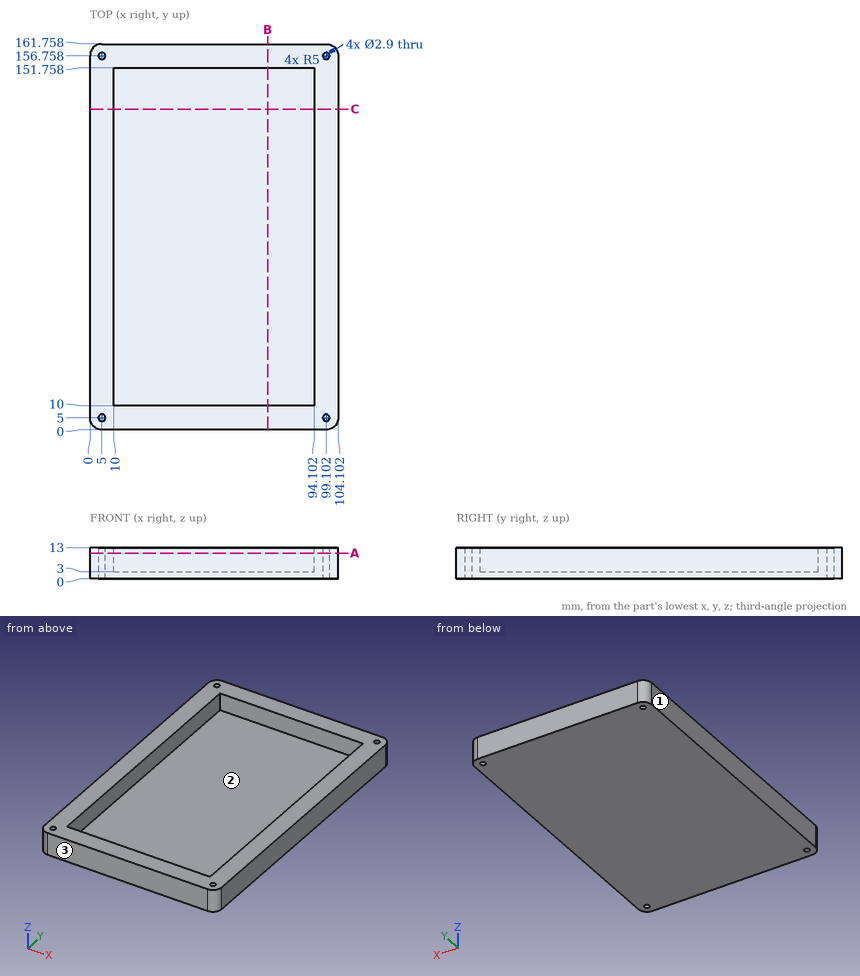
Input: dimensioned drawing with shaded views. Units: mm. Origin: part minimum x, y, z. Coordinates: 2 decimals unless noted, no trailing zeros. Order: outer loops, then holes, each group sorted by start corner. A loop starts at its lowest first (then second) coordinate and runs counter-clockwise, first axis right, second up.
Item 1: Draft query along Y for the marked faces 1, 2 and 3. Return one class per face: released by +Y, released by -Y, zero draft, split by the parting line, or undercut.
Answer:
face 1: zero draft
face 2: undercut
face 3: released by -Y
Item 2: Material intervals for line 1 along Y through (x, z) = (5, 5); line 2 along X through (y, z) = (113, 12.75); line 3 along Y through (x, z) = (77, 11.25), sorted ascending.
Answer:
line 1: y = 0 to 3.55, 6.45 to 155.31, 158.21 to 161.76
line 2: x = 0 to 10, 94.1 to 104.1
line 3: y = 0 to 10, 151.76 to 161.76
Item 3: Section query C-C (y = 134.5). Output: boundary loops of the cut face in (x, z), then the cut area to 3 significant figures.
Answer:
outline: (0, 0) - (104.1, 0) - (104.1, 13) - (94.1, 13) - (94.1, 3) - (10, 3) - (10, 13) - (0, 13) - close
area: 512 mm2
Item 4: Section query B-B (x = 74.5). Output: boundary loops of the cut face in (y, z), then the cut area to 3 significant figures.
Answer:
outline: (0, 0) - (161.76, 0) - (161.76, 13) - (151.76, 13) - (151.76, 3) - (10, 3) - (10, 13) - (0, 13) - close
area: 685 mm2
Item 5: Section query A-A (z = 10.75). Output: boundary loops of the cut face in (x, y), then the cut area to 3 significant figures.
Answer:
outline: (0, 5) arc R5 ccw to (5, 0) - (99.1, 0) arc R5 ccw to (104.1, 5) - (104.1, 156.76) arc R5 ccw to (99.1, 161.76) - (5, 161.76) arc R5 ccw to (0, 156.76) - close; hole circle Ø2.9 at (5, 5); hole circle Ø2.9 at (5, 156.76); hole (10, 10) - (94.1, 10) - (94.1, 151.76) - (10, 151.76) - close; hole circle Ø2.9 at (99.1, 5); hole circle Ø2.9 at (99.1, 156.76)
area: 4,870 mm2
Item 6: Contact query for a flat-ended pin moving along its axis: P1, Ø10, axis at x = 34.5, y = 76.5, coming from the +Z side. Output: stop coordinate, or through.
Answer:
P1: stops at z = 3
